Drawing for the job (mm, zero at the part's lowest x, y, z). A direction names the side the tool comes from. Give positions to 0.01 mm unless a question says otherwise; leave off trailing zeros. Loops run counter-clockwise (first coordinate to the right, second up) from the corner with the lowest first, then second, coordinate; pieces in that order, holes last. Notation, with made-up numbers: (3, 33) -> (60, 33) arc R33 cw to (60, 72) -> close; hole circle Ø4 at (-7.5, -16). An arc over 180 degrees is marked (long way). Write item = value, one per line.
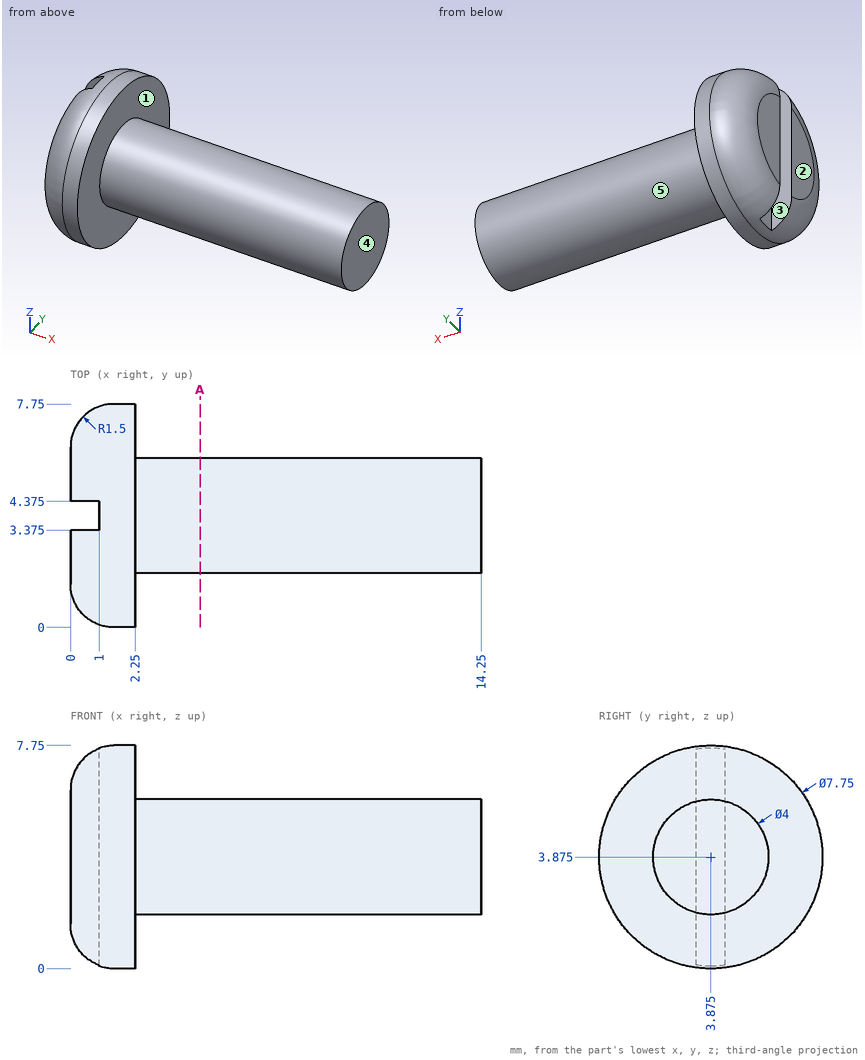
1) Drill centre lines: line 1 along X through (y, z) = (3.75, 1); line 2 along X through (y, z) = (2.75, 5.75); line 3 along Y through (x, z) = (4.75, 3.75). Where is each one in solid material? Low to high. Write a range as [from, to].
Resolved:
line_1 = [1, 2.25]
line_2 = [0, 2.25]
line_3 = [1.88, 5.87]
2) Drop flat-ended pins along their axis: P1, Ø0.8, axis at x = 0.5, z = 2, coming from the +Y side; P2, Ø0.5, axis at x = 0.5, z = 5.5, coming from the -Y side; P3, Ø1, axis at x = 5.5, z = 4.5, coming from the -Y side; P4, Ø1, axis at x = 3, z = 6.5, coming from the +Y side. Give the stop position or say it passes through.
Resolved:
P1 = 7.21
P2 = 0.54
P3 = 1.88
P4 = through
3) Pull direction Y, two halves, no side cores. Call the marked faces 3, 4 and 5: pulls with the +Y half, pulls with the -Y half, needs draft (parallel to the pull), parting line crosses it, or undercut.
Resolved:
face_3 = undercut
face_4 = needs draft
face_5 = parting line crosses it
4) Slice it at A-A, the plane x = 4.5. List the corners of the cut face in (y, z) (3 decimals), and give its area (3 significant figures).
Resolved:
outline = circle Ø4 at (3.875, 3.875)
area = 12.6 mm²
5) Which spindle directions (+Z, -Z, +X, -X, +Y, -Y) get a long thin tool onto all of the face, cutting with end or side? Do the marked faces 1 and 2. Say none if no direction does.
Resolved:
face_1 = +X
face_2 = +Z, -Z, -X, +Y, -Y
